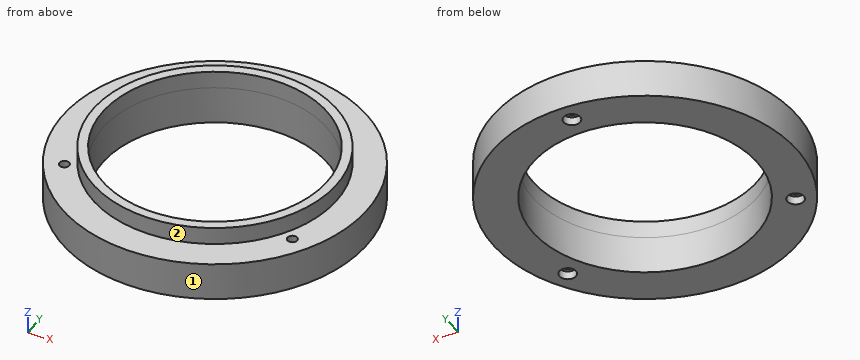
from build123d import *

# Parameters (mm, degrees)
SKETCH1_R           = 50.8
BOSS_EXTRUDE1_DEPTH = 12.7
SKETCH2_R           = 40.64
SKETCH2_R_2         = 37.465
BOSS_EXTRUDE2_DEPTH = 5.842
SKETCH4_R           = 37.465
CUT_EXTRUDE1_DEPTH  = 13.7
CIRPATTERN1_COUNT   = 3


with BuildPart() as part:
    # Sketch1 → Boss-Extrude1 (new body)
    with BuildSketch(Plane.XY):
        Circle(SKETCH1_R)
    extrude(amount=BOSS_EXTRUDE1_DEPTH)

    # Sketch2 → Boss-Extrude2 (add)
    with BuildSketch(Plane.XY.offset(12.7)):
        Circle(SKETCH2_R)
        Circle(SKETCH2_R_2, mode=Mode.SUBTRACT)
    extrude(amount=BOSS_EXTRUDE2_DEPTH)

    # Sketch4 → Cut-Extrude1 (cut, through all)
    with BuildSketch(Plane.XY.offset(12.7)):
        Circle(SKETCH4_R)
    extrude(amount=-CUT_EXTRUDE1_DEPTH, mode=Mode.SUBTRACT)

    # Sketch6 → CBORE for #4 Socket Head Cap Screw1 (revolve, cut)
    with BuildSketch(Plane(origin=(0, 44.45, 0), x_dir=(0, 1, 0), z_dir=(1, 0, 0))):
        Polygon((0, 0), (0, 13.807574487), (1.63195, 12.827), (1.63195, 2.8448), (2.77876, 2.8448), (2.77876, 0), align=None)
    cbore_for_4_socket_head_cap_screw1 = revolve(axis=Axis((0, 44.45, -6.35), (0, 0, 1)), mode=Mode.SUBTRACT)

    # CirPattern1: CBORE for #4 Socket Head Cap Screw1 ×3 about axis
    cirpattern1_axis = Axis((0, 0, 0), (0, 0, 1))
    for i in range(1, CIRPATTERN1_COUNT):
        add(cbore_for_4_socket_head_cap_screw1.rotate(cirpattern1_axis, i * 360 / CIRPATTERN1_COUNT), mode=Mode.SUBTRACT)


solid = part.part
Input: part model. Units: mm. Frame: model coordinates. Face numbers are marked on the shaded views. A direction names the side the tool comes from. Give positions to 0.01 mm unless a question says otherwise; leave off trailing zeros. Order: outer loops, then holes, each group sorted by start corner. A loop starts at its lowest first (then second) coordinate and runs counter-clockwise, first axis right, second up.
Q1. Section C-C on x = 0. Output: boundary loops of the cut face in (y, z) (3 decimals).
Checked values:
outline: (-50.8, 0) - (-37.465, 0) - (-37.465, 18.542) - (-40.64, 18.542) - (-40.64, 12.7) - (-50.8, 12.7) - close; (37.465, 0) - (41.671, 0) - (41.671, 2.845) - (42.818, 2.845) - (42.818, 12.7) - (40.64, 12.7) - (40.64, 18.542) - (37.465, 18.542) - close; (46.082, 2.845) - (47.229, 2.845) - (47.229, 0) - (50.8, 0) - (50.8, 12.7) - (46.082, 12.7) - close
Q2. Section B-B on x = -22. Output: boundary loops of the cut face in (y, z).
Checked values:
outline: (-45.79, 0) - (-30.33, 0) - (-30.33, 18.54) - (-34.17, 18.54) - (-34.17, 12.7) - (-45.79, 12.7) - close; (30.33, 0) - (45.79, 0) - (45.79, 12.7) - (34.17, 12.7) - (34.17, 18.54) - (30.33, 18.54) - close
Q3. Section D-D on y = -39. Output: boundary loops of the cut face in (x, z), and give its area (3 significant figures).
Checked values:
outline: (-32.55, 0) - (32.55, 0) - (32.55, 12.7) - (11.43, 12.7) - (11.43, 18.54) - (-11.43, 18.54) - (-11.43, 12.7) - (-32.55, 12.7) - close
area: 960 mm2
Q4. Section A-A on y = 0. Output: boundary loops of the cut face in (x, z) (3 decimals).
Checked values:
outline: (-50.8, 0) - (-37.465, 0) - (-37.465, 18.542) - (-40.64, 18.542) - (-40.64, 12.7) - (-50.8, 12.7) - close; (37.465, 0) - (50.8, 0) - (50.8, 12.7) - (40.64, 12.7) - (40.64, 18.542) - (37.465, 18.542) - close
Q5. Ray query, probe 1 along Y at (x, z) = (0, 1.65) (3 decimals); probe 2 along Y at (x, z) = (0, 8.75) (3 decimals); probe 3 along X at (y, z) = (-21.5, 7). Return the intervals inside material, ascending.
Checked values:
probe 1: y = -50.8 to -37.465, 37.465 to 41.671, 47.229 to 50.8
probe 2: y = -50.8 to -37.465, 37.465 to 42.818, 46.082 to 50.8
probe 3: x = -46.03 to -39.96, -37.03 to -30.68, 30.68 to 37.03, 39.96 to 46.03
Q6. Contact query for flat-ended pins moving along their axis: pin 1 Ø5 at (x, y) = (-38.49, -22.22) entering from +Z; pin 2 Ø4.5 at (x, y) = (38.49, -22.23) entering from -Z; pin 3 Ø4 at (x, z) = (11.5, 2) entering from +Y; pin 4 Ø2 at (x, y) = (0, 44.45) entering from +Z. Output: stop coordinate, or through.
Checked values:
pin 1: stops at z = 12.7
pin 2: stops at z = 2.84
pin 3: stops at y = 49.9
pin 4: passes through
Q7. Set-up query: the marked faces 1 and 2. Return all of +Z, -Z, +X, -X, +Y, -Y with unobstructed straight access to the full face (end or side cutting, diameter ignored); none if empty.
Checked values:
face 1: +Z, -Z
face 2: +Z
